Geometry check sheet. Reference: the model listing, model coordinates, mm. A direction names the side the tool comes from. Give positions to 0.01 mm unless a question says otherwise; leave off trailing zeros. Order: outer loops, then holes, each group sorted by start corner. A loop starts at its lowest first (then second) coordinate and runs counter-clockwise, first axis right, second up.
from build123d import *

# Parameters (mm, degrees)
EXTRUDE_THIN1_DEPTH = 7.5
BOSS_EXTRUDE1_DEPTH = 3
BOSS_EXTRUDE2_DEPTH = 0.3
LPATTERN1_COUNT     = 4
LPATTERN1_PITCH     = 2.5


with BuildPart() as part:
    # Sketch1 → Extrude-Thin1 (new body)
    with BuildSketch(Plane.XY):
        Polygon((0, 0), (11.7, 0), (11.7, 3.585786438), (10.285786438, 5), (1.414213562, 5), (0, 3.585786438), align=None)
        Polygon((0.5, 0.5), (11.2, 0.5), (11.2, 3.378679656), (10.078679656, 4.5), (1.621320344, 4.5), (0.5, 3.378679656), align=None, mode=Mode.SUBTRACT)
    extrude(amount=EXTRUDE_THIN1_DEPTH)

    # Sketch2 → Boss-Extrude1 (add)
    with BuildSketch(Plane(origin=(0, 0, 0), x_dir=(-1, 0, 0), z_dir=(0, 0, -1))):
        Polygon((0, 0), (0, 3.585786438), (-1.414213562, 5), (-10.285786438, 5), (-11.7, 3.585786438), (-11.7, 0), align=None)
    extrude(amount=-BOSS_EXTRUDE1_DEPTH)

    # Sketch3 → Boss-Extrude2 (add, symmetric)
    with BuildSketch(Plane(origin=(9.6, 0, 0), x_dir=(0, 0, -1), z_dir=(1, 0, 0))):
        with BuildLine():
            Line((-6.5, 2.875), (0, 2.875))
            Line((0, 2.875), (0, -1.8))
            ThreePointArc((0, -1.8), (-0.3, -2.1), (-0.6, -1.8))
            Line((-0.6, -1.8), (-0.6, 2.125))
            Line((-0.6, 2.125), (-6.5, 2.125))
            Line((-6.5, 2.125), (-6.5, 2.875))
        make_face()
    boss_extrude2 = extrude(amount=BOSS_EXTRUDE2_DEPTH, both=True)

    # LPattern1: Boss-Extrude2 ×4
    with Locations(*[(-i * LPATTERN1_PITCH, 0, 0) for i in range(1, LPATTERN1_COUNT)]):
        add(boss_extrude2)


solid = part.part
Item 1: Sectioned sample at A-A (y = -0.25). Enter the section's corners in (x, z), and give its area (3 significant figures).
Reported:
outline: (1.8, 0) - (2.4, 0) - (2.4, 0.6) - (1.8, 0.6) - close; (4.3, 0) - (4.9, 0) - (4.9, 0.6) - (4.3, 0.6) - close; (6.8, 0) - (7.4, 0) - (7.4, 0.6) - (6.8, 0.6) - close; (9.3, 0) - (9.9, 0) - (9.9, 0.6) - (9.3, 0.6) - close
area: 1.44 mm2
Item 2: Scan lines: L1, parallel to Y at x = 9.5, z = 3.5 (3 decimals); L2, parallel to Y at x = 8, z = 4; L3, parallel to Y at x = 5.25, z = 1. Record each from-to range of solid material in increasing order.
Reported:
L1: y = 0 to 0.5, 2.125 to 2.875, 4.5 to 5
L2: y = 0 to 0.5, 4.5 to 5
L3: y = 0 to 5
Item 3: Sectioned sample at D-D (y = 1.25). Enter the section's corners in (x, z), and give its area (3 significant figures).
Reported:
outline: (0, 0) - (11.7, 0) - (11.7, 7.5) - (11.2, 7.5) - (11.2, 3) - (0.5, 3) - (0.5, 7.5) - (0, 7.5) - close
area: 39.6 mm2
Item 4: Gauge pin test, flat ends, axial feed: pin 1 (0.7 mm diameter, centred on x = 9.5, y = -0.5, fed in from +Z); pin 2 (0.7 mm diameter, centred on y = -0.5, z = 0, fed in from -X). Record the tip position at first contact, or that the pin passes through.
Reported:
pin 1: stops at z = 0.6
pin 2: stops at x = 1.8
Item 5: Sectioned sample at B-B (z = 6). Enter the section's corners in (x, y) (3 decimals), and give its area (3 significant figures).
Reported:
outline: (0, 0) - (11.7, 0) - (11.7, 3.586) - (10.286, 5) - (1.414, 5) - (0, 3.586) - close; (1.8, 2.125) - (2.4, 2.125) - (2.4, 2.875) - (1.8, 2.875) - close; (4.3, 2.125) - (4.9, 2.125) - (4.9, 2.875) - (4.3, 2.875) - close; (6.8, 2.125) - (7.4, 2.125) - (7.4, 2.875) - (6.8, 2.875) - close; (9.3, 2.125) - (9.9, 2.125) - (9.9, 2.875) - (9.3, 2.875) - close; hole (0.5, 0.5) - (11.2, 0.5) - (11.2, 3.379) - (10.079, 4.5) - (1.621, 4.5) - (0.5, 3.379) - close
area: 16.8 mm2
Item 6: Sectioned sample at C-C (x = 7). Enter the section's corners in (y, z) (3 decimals).
Reported:
outline: (-1.8, 0) - (5, 0) - (5, 7.5) - (4.5, 7.5) - (4.5, 3) - (2.875, 3) - (2.875, 6.5) - (2.125, 6.5) - (2.125, 3) - (0.5, 3) - (0.5, 7.5) - (0, 7.5) - (0, 0.6) - (-1.8, 0.6) arc R0.3 ccw to start
Item 7: Draft check along X on faces 1 (the flat face through (11.003, 4.283, 3.698)), 2 (the flat face through (5.8, 0.3, 7.5)), 3 (the flat face through (1.07, 3.95, 5.22)), 4 (the flat face through (6, 3, 3)). Enter one of: released by +X, released by -X, zero draft, split by the parting line, or undercut.
Reported:
face 1: released by +X
face 2: zero draft
face 3: undercut
face 4: undercut
Item 8: Set-up check for faces 5 (the flat face through (10.65, 3.93, 5.22)), 6 (the flat face through (6, 5, 4)): record each of +Z, -Z, +X, -X, +Y, -Y from which the full face is reachable in a straight line by a thin tool's end or side.
Reported:
face 5: +Z
face 6: +Z, -Z, +X, -X, +Y
